Design review of the part built by this model. Coordinates are the model's own, in mm. Face numbers are marked on the shaded views. A direction names the side the tool comes from. Round coordinates to 2 decimals unless told otherwise and drop trailing zeros. Loops run counter-clockwise (first coordinate to the right, second up) from the corner with the lowest first, then second, coordinate; pieces in that order, holes last. Notation, with made-up numbers: M 55,-13 L 75,-13 A19 ccw 75,-5 Z; hole C 74.5,-15 d6. An arc over 180 degrees is marked long. Use a Markdown table: item, result.
from build123d import *

# Parameters (mm, degrees)
ESQUISSE1_W             = 52
ESQUISSE1_H             = 202
BOSS_EXTRU_1_DEPTH      = 102
COQUE1_T                = -1
ESQUISSE2_W             = 50
ESQUISSE2_H             = 200
BOSS_EXTRU_2_DEPTH      = 1
ESQUISSE3_R             = 5.5
ENL_V_MAT_EXTRU_1_DEPTH = 1
ESQUISSE4_W             = 1
ESQUISSE4_H             = 202
BOSS_EXTRU_3_DEPTH      = 20


with BuildPart() as part:
    # Esquisse1 → Boss.-Extru.1 (new body)
    with BuildSketch(Plane.XY):
        Rectangle(ESQUISSE1_W, ESQUISSE1_H)
    extrude(amount=BOSS_EXTRU_1_DEPTH)

    # Coque1
    coque1_openings = [part.faces().sort_by_distance(p)[0] for p in [
        (0, 0, 102),
    ]]
    offset(amount=COQUE1_T, openings=coque1_openings, kind=Kind.INTERSECTION)

    # Esquisse2 → Boss.-Extru.2 (add)
    with BuildSketch(Plane.XY.offset(102)):
        Rectangle(ESQUISSE2_W, ESQUISSE2_H)
    extrude(amount=-BOSS_EXTRU_2_DEPTH)

    # Esquisse3 → Enlèv. mat.-Extru.1 (cut)
    with BuildSketch(Plane.XY.offset(102)):
        with Locations((0, -81)):
            Circle(ESQUISSE3_R)
        with Locations((0, -51)):
            Circle(ESQUISSE3_R)
    extrude(amount=-ENL_V_MAT_EXTRU_1_DEPTH, mode=Mode.SUBTRACT)

    # Esquisse4 → Boss.-Extru.3 (add)
    with BuildSketch(Plane(origin=(26, 0, 0), x_dir=(0, 0, -1), z_dir=(1, 0, 0))):
        with Locations((-0.5, 0)):
            Rectangle(ESQUISSE4_W, ESQUISSE4_H)
    extrude(amount=BOSS_EXTRU_3_DEPTH)


solid = part.part
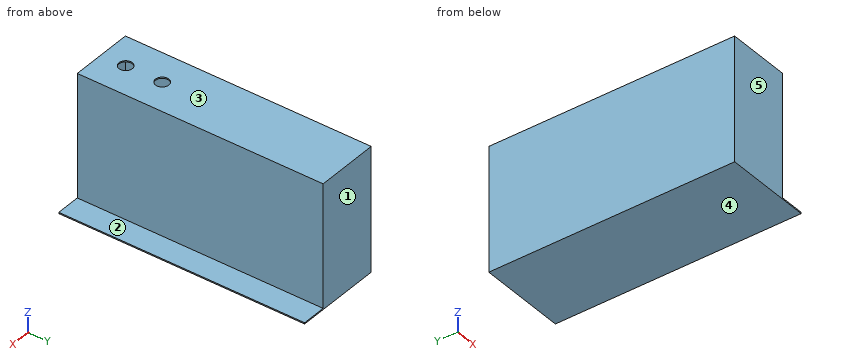
1. Take a section at C-C on y = 26. Give the boundary of the cut face in (x, z), and give its area (3 significant figures).
Check values:
| item | result |
|---|---|
| outline | M -26,0 L 46,0 L 46,1 L 26,1 L 26,102 L -26,102 Z; hole M -25,1 L 25,1 L 25,101 L -25,101 Z |
| area | 324 mm² |
2. Take a section at B-B on z = 57. Give the boundary of the cut face in (x, y), and give its area (3 significant figures).
Check values:
| item | result |
|---|---|
| outline | M -26,-101 L 26,-101 L 26,101 L -26,101 Z; hole M -25,-100 L 25,-100 L 25,100 L -25,100 Z |
| area | 504 mm² |
3. Take a section at D-D on y = -81. Give the boundary of the cut face in (x, z), and give its area (3 significant figures).
Check values:
| item | result |
|---|---|
| outline | M -26,0 L 46,0 L 46,1 L 26,1 L 26,102 L 5.5,102 L 5.5,101 L 25,101 L 25,1 L -25,1 L -25,101 L -5.5,101 L -5.5,102 L -26,102 Z |
| area | 313 mm² |
4. Insertion check: pin 1 (6.5 mm diameter, centred on x = 0, y = -51, fed in from +Z); pin 2 (6 mm diameter, centred on y = -78, z = 42.5, fed in from +X); pin 3 (10 mm diameter, centred on x = 34, z = 51, fed in from +Y). Each pin has a flat end and moves straight along its axis. Give the tip position at first contact, or say it passes through.
Check values:
| item | result |
|---|---|
| pin 1 | stops at z = 1 |
| pin 2 | stops at x = 26 |
| pin 3 | passes through |
5. Wall thickness on line 1 along Y through (x, z) = (0, 101.4); line 2 along Z through (x, y) = (3.5, -61); line 3 along X through (y, z) = (-43, 9): over which ranges is each line inside the solid? List them lowest first. Write a range as from..to.
Check values:
| item | result |
|---|---|
| line 1 | y = -101..-86.5, -75.5..-56.5, -45.5..101 |
| line 2 | z = 0..1, 101..102 |
| line 3 | x = -26..-25, 25..26 |
6. Machinability: for the marked faces 1 and 2, which of the approach directions +Z, -Z, +X, -X, +Y, -Y give a long, thin tool a straight path to every point of the face, cutting with its end or side? Answer none if there is none.
Check values:
| item | result |
|---|---|
| face 1 | +Z, -Z, +X, -X, +Y |
| face 2 | +Z, +X, +Y, -Y |
7. The part is to be moulded in two halves that separate along Z. For the marked faces 3, 4 and 5, say which applies: pulls with the +Z half, pulls with the -Z half, needs draft (parallel to the pull), parting line crosses it, or undercut.
Check values:
| item | result |
|---|---|
| face 3 | pulls with the +Z half |
| face 4 | pulls with the -Z half |
| face 5 | needs draft |
8. Take a section at A-A on x = 0. Give the boundary of the cut face in (y, z).
Check values:
| item | result |
|---|---|
| outline | M -101,0 L 101,0 L 101,102 L -45.5,102 L -45.5,101 L 100,101 L 100,1 L -100,1 L -100,101 L -86.5,101 L -86.5,102 L -101,102 Z; M -75.5,101 L -56.5,101 L -56.5,102 L -75.5,102 Z |
